Could you check a few things on this model? Use its own coordinates, in mm. Face numbers are marked on the shaded views. A direction names the side the tool comes from. Coordinates: 2 decimals unless noted, no trailing zeros. Write each loop counter-clockwise with the first axis right and the second up, starting at its lowest first coordinate (ties: lowest second). Pieces come first, ordered by that corner, then holes.
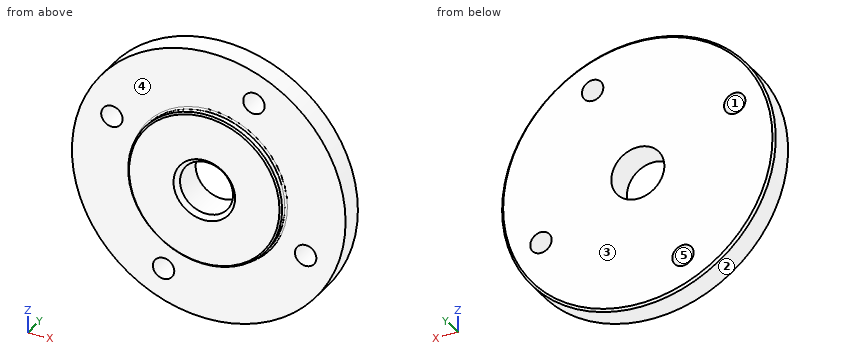
```python
from build123d import *

# Parameters (mm, degrees)
CHANFRO1_SIZE                 = 0.5
FURO_ROSCADO_DE_M3X0_52_D     = 2.5
FURO_ROSCADO_DE_M3X0_52_DEPTH = 3.001
PADR_OCIRCULAR2_COUNT         = 4
CHANFRO2_SIZE                 = 0.2
CHANFRO3_SIZE                 = 0.25
FILETE3_R                     = 0.2


with BuildPart() as part:
    # Esboço1 → Revolução1 (revolve)
    with BuildSketch(Plane.XY):
        Polygon((3.1, 1.5), (3.1, -2.5), (9, -2.5), (9, -1.5), (16, -1.5), (16, 1.5), align=None)
    revolve(axis=Axis((0, 0, 0), (0, 1, 0)))

    # Chanfro1
    chanfro1_edges = [part.edges().sort_by_distance(p)[0] for p in [
        (-3.1, -2.5, 0),
    ]]
    chamfer(chanfro1_edges, length=CHANFRO1_SIZE)

    # Furo roscado de M3x0.52
    with Locations(Plane(origin=(0, 1.5, 0), x_dir=(1, 0, 0), z_dir=(0, 1, 0))):
        with Locations((11.328847338, 5.282728272)):
            furo_roscado_de_m3x0_52 = Hole(FURO_ROSCADO_DE_M3X0_52_D / 2, depth=FURO_ROSCADO_DE_M3X0_52_DEPTH)

    # PadrãoCircular2: Furo roscado de M3x0.52 ×4 about axis
    padr_ocircular2_axis = Axis((0, 0, 0), (0, 1, 0))
    for i in range(1, PADR_OCIRCULAR2_COUNT):
        add(furo_roscado_de_m3x0_52.rotate(padr_ocircular2_axis, i * 360 / PADR_OCIRCULAR2_COUNT), mode=Mode.SUBTRACT)

    # Chanfro2
    chanfro2_edges = [part.edges().sort_by_distance(p)[0] for p in [
        (-9, -2.5, 0),
    ]]
    chamfer(chanfro2_edges, length=CHANFRO2_SIZE)

    # Chanfro3
    chanfro3_edges = [part.edges().sort_by_distance(p)[0] for p in [
        (-16, 1.5, 0),
    ]]
    chamfer(chanfro3_edges, length=CHANFRO3_SIZE)

    # Filete3
    filete3_edges = [part.edges().sort_by_distance(p)[0] for p in [
        (-9, -1.5, 0),
    ]]
    fillet(filete3_edges, radius=FILETE3_R)


solid = part.part
```
1. For pin 1 (2 mm diameter, centred on x = 7.5, y = 0, fed in from +Z); pin 2 (3 mm diameter, centred on x = 11.5, z = 7, fed in from -Y); pin 3 (1.5 mm diameter, centred on x = -11.33, z = 5.28, fed in from -Y); pin 4 (1.5 mm diameter, centred on y = 1, z = -1, fed in from +X), each with a flat end and sliding along its axis, tell me the tip position at first contact or that it passes through.
Verdict:
pin 1: stops at z = 14.62
pin 2: stops at y = -1.5
pin 3: passes through
pin 4: stops at x = 16
2. I want a section at A-A on x = 0. Please give me the cut outline in (y, z).
Verdict:
outline: (-2.5, -8.8) - (-2.3, -9) - (-1.7, -9) arc R0.2 cw to (-1.5, -9.2) - (-1.5, -16) - (1.25, -16) - (1.5, -15.75) - (1.5, -3.1) - (-2, -3.1) - (-2.5, -3.6) - close; (-2.5, 3.6) - (-2, 3.1) - (1.5, 3.1) - (1.5, 15.75) - (1.25, 16) - (-1.5, 16) - (-1.5, 9.2) arc R0.2 cw to (-1.7, 9) - (-2.3, 9) - (-2.5, 8.8) - close
3. If we mould it in two halves opening along Z, with no side actions, what happens to the marked faces 1, 2 and 3? For each: pulls with the +Z half, pulls with the -Z half, needs draft (parallel to the pull), parting line crosses it, or undercut.
Verdict:
face 1: undercut
face 2: parting line crosses it
face 3: needs draft
4. I want a section at B-B on z = 0. Please give me the cut outline in (x, y).
Verdict:
outline: (-16, -1.5) - (-9.2, -1.5) arc R0.2 cw to (-9, -1.7) - (-9, -2.3) - (-8.8, -2.5) - (-3.6, -2.5) - (-3.1, -2) - (-3.1, 1.5) - (-15.75, 1.5) - (-16, 1.25) - close; (3.1, -2) - (3.6, -2.5) - (8.8, -2.5) - (9, -2.3) - (9, -1.7) arc R0.2 cw to (9.2, -1.5) - (16, -1.5) - (16, 1.25) - (15.75, 1.5) - (3.1, 1.5) - close
5. On a 3-axis mill with a long thin cutter (end or side, diameter ignored), from which of +Z, -Z, +X, -X, +Y, -Y can I reach the whole of each face in a straight line? I mean the marked faces 4 and 5. Say none if no direction works.
Verdict:
face 4: -Y
face 5: +Y, -Y
6. I want a section at C-C on y = 0.35. Please give me the cut outline in (x, z), plus the area to 3 significant figures.
Verdict:
outline: circle Ø32 at (0, 0); hole circle Ø2.5 at (-11.33, 5.28); hole circle Ø2.5 at (-5.28, -11.33); hole circle Ø6.2 at (0, 0); hole circle Ø2.5 at (5.28, 11.33); hole circle Ø2.5 at (11.33, -5.28)
area: 754 mm2
7. Please list where these lines run through material, in increasing order: line 1 along X through (y, z) = (0.7, 0); line 2 along Y through (x, z) = (9, -10); line 3 along X through (y, z) = (0.3, -1.5).
Verdict:
line 1: x = -16 to -3.1, 3.1 to 16
line 2: y = -1.5 to 1.5
line 3: x = -15.93 to -2.71, 2.71 to 15.93
